from build123d import *

# Parameters (mm, degrees)
SKETCH1_R              = 38.1
SKETCH1_R_2            = 9.525
BOSS_EXTRUDE1_DEPTH    = 38.1
F_10_32_TAPPED_HOLE1_D = 4.826
CIRPATTERN1_COUNT      = 8
SKETCH4_W              = 6.35
SKETCH4_H              = 6.35
CUT_EXTRUDE1_DEPTH     = 66.991135768
SKETCH5_W              = 2.0828
SKETCH5_H              = 25.4
SKETCH7_OUTSIDE_W      = 101.06
SKETCH7_OUTSIDE_H      = 101.06
SKETCH7_OUTSIDE_R      = 19.05
CUT_EXTRUDE2_DEPTH     = 28.575
FILLET1_R              = 3.175


with BuildPart() as part:
    # Sketch1 → Boss-Extrude1 (new body)
    with BuildSketch(Plane(origin=(0, 0, 0), x_dir=(1, 0, 0), z_dir=(0, 1, 0))):
        with Locations(Location((0, 0, 0), (0, 0, 90))):
            Circle(SKETCH1_R)
        with Locations(Location((0, 0, 0), (0, 0, 90))):
            Circle(SKETCH1_R_2, mode=Mode.SUBTRACT)
    extrude(amount=BOSS_EXTRUDE1_DEPTH)

    # #10-32 Tapped Hole1 (through all)
    with Locations(Plane(origin=(0, 38.1, 0), x_dir=(-1, 0, 0), z_dir=(0, 1, 0))):
        with Locations((29.333175157, -12.150198978)):
            f_10_32_tapped_hole1 = Hole(F_10_32_TAPPED_HOLE1_D / 2)

    # CirPattern1: #10-32 Tapped Hole1 ×8 about axis
    cirpattern1_axis = Axis((0, 0, 0), (0, 1, 0))
    for i in range(1, CIRPATTERN1_COUNT):
        add(f_10_32_tapped_hole1.rotate(cirpattern1_axis, i * 360 / CIRPATTERN1_COUNT), mode=Mode.SUBTRACT)

    # Sketch4 → Cut-Extrude1 (cut, through all)
    with BuildSketch(Plane(origin=(0, 38.1, 0), x_dir=(1, 0, 0), z_dir=(0, 1, 0))):
        with Locations((0, -9.525)):
            Rectangle(SKETCH4_W, SKETCH4_H)
    extrude(amount=-CUT_EXTRUDE1_DEPTH, mode=Mode.SUBTRACT)

    # Sketch5 → #8-32 Tapped Hole1 (revolve, cut)
    with BuildSketch(Plane(origin=(0, 19.05, 12.7), x_dir=(0, 1, 0), z_dir=(1, 0, 0))):
        with Locations((1.0414, 12.7)):
            Rectangle(SKETCH5_W, SKETCH5_H)
    revolve(axis=Axis((0, 19.05, 6.35), (0, 0, 1)), mode=Mode.SUBTRACT)

    # Sketch7 outside → Cut-Extrude2 (cut)
    with BuildSketch(Plane(origin=(0, 38.1, 0), x_dir=(1, 0, 0), z_dir=(0, 1, 0))):
        Rectangle(SKETCH7_OUTSIDE_W, SKETCH7_OUTSIDE_H)
        with Locations(Location((0, 0, 0), (0, 0, 270))):
            Circle(SKETCH7_OUTSIDE_R, mode=Mode.SUBTRACT)
    extrude(amount=-CUT_EXTRUDE2_DEPTH, mode=Mode.SUBTRACT)

    # Fillet1
    fillet1_edges = [part.edges().sort_by_distance(p)[0] for p in [
        (0, 9.525, -19.05),
    ]]
    fillet(fillet1_edges, radius=FILLET1_R)


solid = part.part
Check sheet for the modelled part. Datum: model origin and axes. Units: mm. A direction names the side the tool comes from. Give positions to 0.01 mm unless a question says otherwise; leave off trailing zeros. Write each loop counter-clockwise with the first axis right and the second up, starting at its lowest first coordinate (ties: lowest second). Pieces come first, ordered by that corner, then holes. Notation, with made-up numbers: (81.25, 52) -> (140.25, 52) arc R37 ccw to (140.25, 89) -> close; hole circle Ø9 at (12.25, 48.5). An arc over 180 degrees is marked (long way). One line per item, written item: value. Start each with the question number.
Item 1: Section check B-B on x = 0. Record the cut outline in (y, z) (3 decimals), then the cut area to 3 significant figures.
Item 2: Gauge pin test, flat ends, axial feed: pin 1 (7.5 mm diameter, centred on x = 29.33, z = 12.15, fed in from +Y) (3 decimals); pin 2 (4 mm diameter, centred on y = 23, z = 12, fed in from +X); pin 3 (3 mm diameter, centred on y = 18, z = 5, fed in from -X). Record the tip position at first contact, or that the pin passes through.
Item 3: Section check A-A on z = 0. Record the cut outline in (x, y) (3 decimals).
Item 4: Section check D-D on y = 19.05. Record the cut outline in (x, z) (3 decimals).
Item 5: Section check C-C on y = 15. Record the cut outline in (x, z) (3 decimals).
Item 6: Draft check along Z on faces 1 (the cylindrical face through (31.744, 4.696, 12.044)), 2 (the cylindrical face through (-31.725, 4.696, 12.466)), 3 (the cylindrical face through (23.183, 4.696, 30.235)), 4 (the cylindrical face through (1.27, 17.4, 15.92)). Enter one of: +Z half, -Z half, draft (parallel to the pull), parting line (faces both ways), or undercut.
Item 7: Tool access check on faces 5 (the cylindrical face through (-11.59, 25.58, -15.12)), 6 (the flat face through (4, 38.1, 9)), 7 (the flat face through (-3.175, 19, 11)). Record the directions out of +Z, -Z, +X, -X, +Y, -Y that give a thin tool (end or side, any length) a straight path to the whole face; none if there is none.
Item 8: Material ranges on probe 1 along Y at (x, z) = (32.5, 3) (3 decimals); probe 2 along Y at (x, z) = (0, 14.5); probe 3 along X at (y, z) = (20.5, 15.5), recorded low to high. Write a range as from..to.
Results list:
1. outline: (0, -38.1) -> (9.525, -38.1) -> (9.525, -22.225) arc R3.175 cw to (12.7, -19.05) -> (38.1, -19.05) -> (38.1, -9.525) -> (0, -9.525) -> close; (0, 12.7) -> (16.967, 12.7) -> (16.967, 19.05) -> (12.7, 19.05) arc R3.175 cw to (9.525, 22.225) -> (9.525, 38.1) -> (0, 38.1) -> close; (21.133, 12.7) -> (38.1, 12.7) -> (38.1, 19.05) -> (21.133, 19.05) -> close
1. area: 946 mm²
2. pin 1: y = 9.525
2. pin 2: x = 16.21
2. pin 3: x = -18.73
3. outline: (-38.1, 0) -> (-9.525, 0) -> (-9.525, 38.1) -> (-19.05, 38.1) -> (-19.05, 12.7) arc R3.175 cw to (-22.225, 9.525) -> (-38.1, 9.525) -> close; (9.525, 0) -> (38.1, 0) -> (38.1, 9.525) -> (22.225, 9.525) arc R3.175 cw to (19.05, 12.7) -> (19.05, 38.1) -> (9.525, 38.1) -> close
4. outline: (-3.175, 8.98) -> (-3.175, 12.7) -> (-2.083, 12.7) -> (-2.083, 18.936) arc R19.05 ccw (long way) to (2.083, 18.936) -> (2.083, 12.7) -> (3.175, 12.7) -> (3.175, 8.98) arc R9.525 cw (long way) to start
5. outline: circle Ø38.1 at (0, 0); hole (-3.175, 8.98) arc R9.525 ccw (long way) to (3.175, 8.98) -> (3.175, 12.7) -> (-3.175, 12.7) -> close
6. face 1: undercut
6. face 2: undercut
6. face 3: parting line
6. face 4: draft
7. face 5: +Y
7. face 6: +Z, -Z, +X, -X, +Y
7. face 7: +Y, -Y
8. probe 1: 0..9.525
8. probe 2: 0..16.97, 21.13..38.1
8. probe 3: -11.07..-1.5, 1.5..11.07
